Geometry check sheet. Reference: the model listing, model coordinates, mm. Face numbers are marked on the shaded views. A direction names the side the tool comes from. Give positions to 0.01 mm unless a question says otherwise; leave off trailing zeros. Write each loop counter-clockwise with the first axis right and the second up, starting at its lowest first coordinate (ties: lowest second). Pieces come first, ordered by that corner, then holes.
(1) Thickness scan on line 1 along Y through (x, z) = (-22, -39.5). Record the ranges inside material, lowest first.
(2) Cross-section at A-A (z = 1). Record the boundary of the cut face in (x, y).
(3) Tool access check on the marked faces 1, 2, 3 and 4. Record the directions out of +Z, -Z, +X, -X, +Y, -Y that give a thin tool (end or side, any length) a straight path to the whole face; none if there is none.
(4) Cross-section at B-B (y = 14). Record the boundary of the cut face in (x, z).
(5) Mould release check, pull along Z, two halves, no side actions. Record for the marked faces 5, 6, 7 and 8: +Z half, -Z half, draft (parallel to the pull), parting line (faces both ways), or undercut.
(6) Depth check by flat-ended pin: P1, Ø4, axis at y = -1.5, z = 29, coming from the +X side; P2, Ø6.5, axis at x = -3, z = -36, coming from the +Y side; P3, Ø1, axis at x = 4, z = -34, coming from the -Y side. Enter the tip coordinate at first touch or a pass-through.
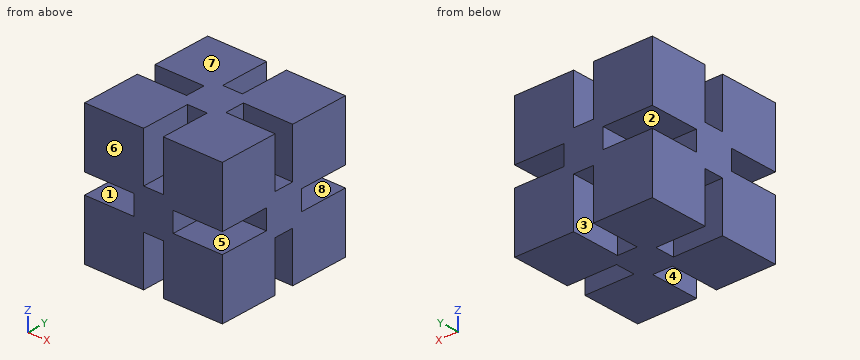
```python
from build123d import *

# Parameters (mm, degrees)
F0_W     = 88.9
F0_H     = 88.9
F1_DEPTH = 44.45
F2_W     = 35.494227
F2_H     = 12.7
F2_W_2   = 12.7
F2_H_2   = 43.843563
F2_W_3   = 49.659715
F2_H_3   = 53.186459
F3_DEPTH = 31.75
F4_W     = 43.534182
F4_H     = 12.7
F4_W_2   = 12.7
F4_H_2   = 43.534182
F5_DEPTH = 31.75
F6_W     = 39.738709
F6_H     = 12.7
F6_W_2   = 51.209684
F7_DEPTH = 31.75
F8_W     = 39.158334
F8_H     = 12.7
F8_W_2   = 39.793333
F9_DEPTH = 31.75


with BuildPart() as f1:
    # F0 (on Top) → F1 (new body, symmetric)
    with BuildSketch(Plane.XY):
        Rectangle(F0_W, F0_H)
    extrude(amount=F1_DEPTH, both=True)

    # F2 (on face) → F3 (cut)
    with BuildSketch(Plane.XY.offset(44.45)):
        with Locations((30.447114, 0)):
            Rectangle(F2_W, F2_H)
        with Locations((0, -34.621781)):
            Rectangle(F2_W_2, F2_H_2)
        with Locations((-37.529857, 0)):
            Rectangle(F2_W_3, F2_H)
        with Locations((0, 39.29323)):
            Rectangle(F2_W_2, F2_H_3)
    extrude(amount=-F3_DEPTH, mode=Mode.SUBTRACT)

    # F4 (on face) → F5 (cut)
    with BuildSketch(Plane(origin=(0, 0, -44.45), x_dir=(1, 0, 0), z_dir=(0, 0, -1))):
        with Locations((34.467091, 0)):
            Rectangle(F4_W, F4_H)
        with Locations((0, 34.467091)):
            Rectangle(F4_W_2, F4_H_2)
        with Locations((-34.467091, 0)):
            Rectangle(F4_W, F4_H)
        with Locations((0, -34.467091)):
            Rectangle(F4_W_2, F4_H_2)
    extrude(amount=-F5_DEPTH, mode=Mode.SUBTRACT)

    # F6 (on face) → F7 (cut)
    with BuildSketch(Plane.XZ.offset(44.45)):
        with Locations((32.569354, 0)):
            Rectangle(F6_W, F6_H)
        with Locations((-38.304842, 0)):
            Rectangle(F6_W_2, F6_H)
    extrude(amount=-F7_DEPTH, mode=Mode.SUBTRACT)

    # F8 (on face) → F9 (cut)
    with BuildSketch(Plane(origin=(0, 44.45, 0), x_dir=(-1, 0, 0), z_dir=(0, 1, 0))):
        with Locations((32.279167, 0)):
            Rectangle(F8_W, F8_H)
        with Locations((-32.596666, 0)):
            Rectangle(F8_W_2, F8_H)
    extrude(amount=-F9_DEPTH, mode=Mode.SUBTRACT)


solid = f1.part
```
Reply:
1. line 1: y = -44.45 to -6.35, 6.35 to 44.45
2. outline: (-44.45, -12.7) - (-12.7, -12.7) - (-12.7, -44.45) - (12.7, -44.45) - (12.7, -12.7) - (44.45, -12.7) - (44.45, 12.7) - (12.7, 12.7) - (12.7, 44.45) - (-12.7, 44.45) - (-12.7, 12.7) - (-44.45, 12.7) - close
3. face 1: -X, -Y
3. face 2: -X, +Y
3. face 3: -Z, +Y
3. face 4: -Z, -Y
4. outline: (-44.45, -44.45) - (-6.35, -44.45) - (-6.35, -12.7) - (6.35, -12.7) - (6.35, -44.45) - (44.45, -44.45) - (44.45, -6.35) - (12.7, -6.35) - (12.7, 6.35) - (44.45, 6.35) - (44.45, 44.45) - (6.35, 44.45) - (6.35, 12.7) - (-6.35, 12.7) - (-6.35, 44.45) - (-44.45, 44.45) - (-44.45, 6.35) - (-12.7, 6.35) - (-12.7, -6.35) - (-44.45, -6.35) - close
5. face 5: undercut
5. face 6: draft
5. face 7: +Z half
5. face 8: undercut
6. P1: stops at x = 12.7
6. P2: stops at y = 12.7
6. P3: stops at y = -12.7
